Could you check a few things on this drawing? It's one solid part, dimensions in mm from its lowest x, y, z. Coordinates: 2 decimals unless noted, no trailing zeros. Write each loop counter-clockwise with the first axis right and the second up, starting at its lowest first coordinate (ties: lowest second). Pieces come first, ordered by that corner, then holes.
Item 1: If we mould it in two halves opening along X, with no side actions, what happens to the marked faces 1, 2 and 3? For each: pulls with the +X half, pulls with the -X half, needs draft (parallel to the pull), parting line crosses it, or undercut.
Item 2: I want a section at D-D (x = 20.5). Please give me the cut outline in (y, z) (1 decimal), and give its area (3 significant figures).
Item 3: I want a section at C-C (y = 5). Please give me the cut outline in (x, z) (1 decimal), and give its area (3 significant figures).
Item 4: I'm going to push flat-ended pins straight in: P1, Ø1.6, axis at x = 42.5, z = 47.5, coming from the +Y side; P2, Ø1, axis at x = 28.5, y = 1, coming from the +Z side; P3, Ø1.5, axis at x = 59, y = 6, coming from the +Z side. Where does each tip first touch, or does it pass through?
Item 5: I want a section at A-A (x = 35). Please give me the cut outline in (y, z).
Item 6: Please list where these lines run through material, in increasing order: line 1 (Z direction, x = 42, y = 3) (1 decimal); line 2 (Z direction, x = 38, y = 3.5) (1 decimal); line 3 (Z direction, x = 41.5, y = 1).
Item 7: I want a section at B-B (z = 35). Please give me the cut outline in (x, y), and give its area (3 significant figures).
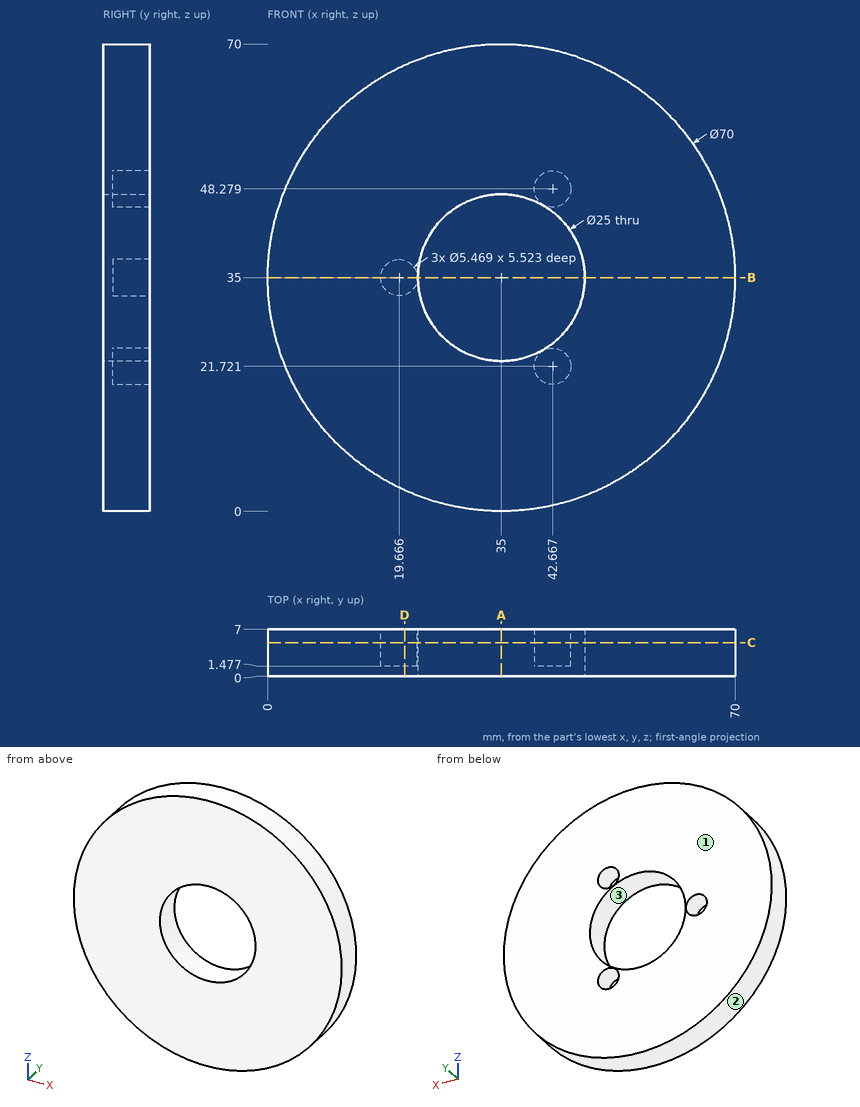
Answer:
1. face 1: needs draft
1. face 2: parting line crosses it
1. face 3: undercut
2. outline: (0, 3.1) - (7, 3.1) - (7, 32.4) - (1.5, 32.4) - (1.5, 37.6) - (7, 37.6) - (7, 66.9) - (0, 66.9) - close
2. area: 417 mm2
3. outline: circle Ø70 at (35, 35); hole circle Ø5.5 at (19.7, 35); hole circle Ø25 at (35, 35); hole circle Ø5.5 at (42.7, 21.7); hole circle Ø5.5 at (42.7, 48.3)
3. area: 3,290 mm2
4. P1: stops at y = 1.48
4. P2: stops at z = 69.48
4. P3: stops at z = 61.16
5. outline: (0, 0) - (7, 0) - (7, 22.5) - (0, 22.5) - close; (0, 47.5) - (7, 47.5) - (7, 70) - (0, 70) - close
6. line 1: z = 0.7 to 19.1, 24.4 to 24.6, 45.4 to 45.6, 50.9 to 69.3
6. line 2: z = 0.1 to 22.9, 47.1 to 69.9
6. line 3: z = 0.61 to 24.32, 45.68 to 69.39
7. outline: (0, 0) - (22.5, 0) - (22.5, 7) - (22.4, 7) - (22.4, 1.48) - (16.93, 1.48) - (16.93, 7) - (0, 7) - close; (47.5, 0) - (70, 0) - (70, 7) - (47.5, 7) - close
7. area: 285 mm2
